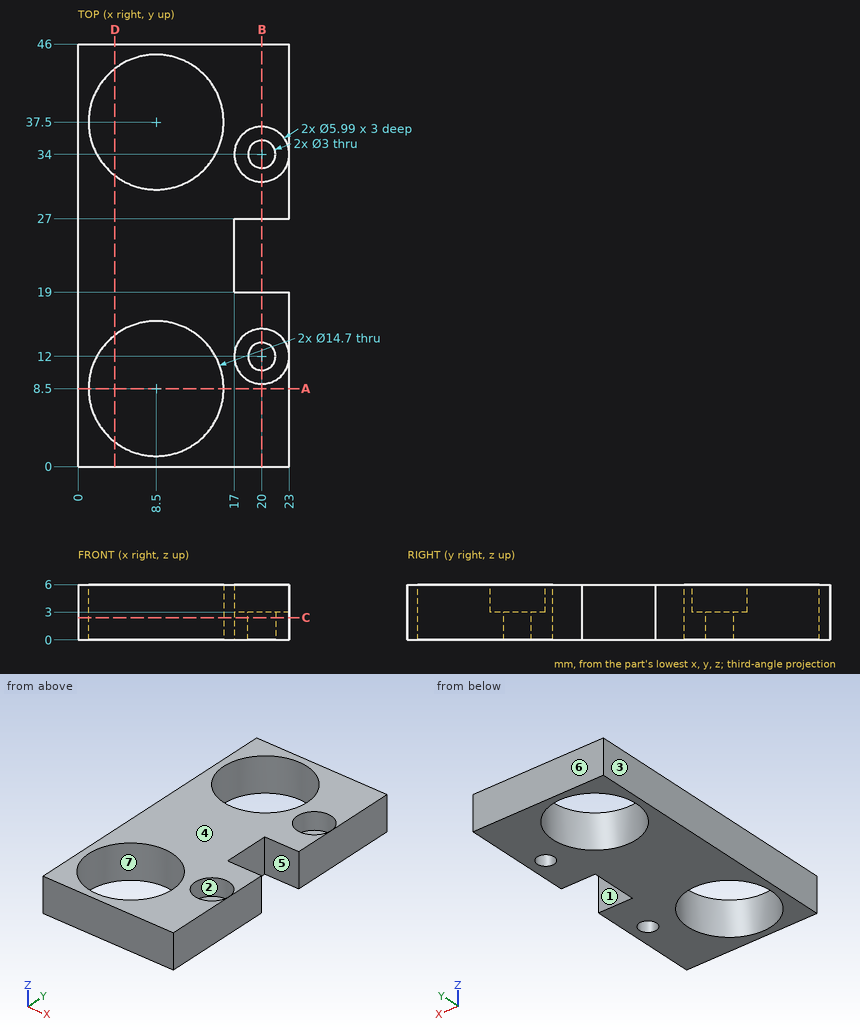
Here's the drawing with two shaded views (mm, measured from the low corner). I have some questions. A direction names the side the tool comes from. Coordinates: 2 decimals unless noted, no trailing zeros. Order: outer loops, then holes, each group sorted by start corner. A loop starts at its lowest first (then second) coordinate and runs counter-clockwise, first axis right, second up. Notation, with made-up numbers: (26.25, 41) - (45.25, 41) arc R30 ccw to (45.25, 76) - close; hole circle Ø10 at (5, 52). An arc over 180 degrees is marked (long way). Answer in a Markdown table with one row per item.
1. Suppose I cut it at C-C (z = 2.4). Please give me the cut outline in (x, y), and give its area (3 significant figures).
Reply:
| item | result |
|---|---|
| outline | (0, 0) - (23, 0) - (23, 19) - (17, 19) - (17, 27) - (23, 27) - (23, 46) - (0, 46) - close; hole circle Ø14.7 at (8.5, 8.5); hole circle Ø14.7 at (8.5, 37.5); hole circle Ø3 at (20, 12); hole circle Ø3 at (20, 34) |
| area | 656 mm^2 |
2. Suppose I cut it at B-B (x = 20). Please give me the cut outline in (y, z) (3 decimals).
Reply:
| item | result |
|---|---|
| outline | (0, 0) - (10.5, 0) - (10.5, 3) - (9.005, 3) - (9.005, 6) - (0, 6) - close; (13.5, 0) - (19, 0) - (19, 6) - (14.995, 6) - (14.995, 3) - (13.5, 3) - close; (27, 0) - (32.5, 0) - (32.5, 3) - (31.005, 3) - (31.005, 6) - (27, 6) - close; (35.5, 0) - (46, 0) - (46, 6) - (36.995, 6) - (36.995, 3) - (35.5, 3) - close |
3. Suppose I cut it at D-D (x = 4). Please give me the cut outline in (y, z).
Reply:
| item | result |
|---|---|
| outline | (0, 0) - (2.69, 0) - (2.69, 6) - (0, 6) - close; (14.31, 0) - (31.69, 0) - (31.69, 6) - (14.31, 6) - close; (43.31, 0) - (46, 0) - (46, 6) - (43.31, 6) - close |
4. If we mould it in two halves opening along Y, with no side actions, what happens to the marked faces 4, 5, 6 and 7? For each: pulls with the +Y half, pulls with the -Y half, needs draft (parallel to the pull), parting line crosses it, or undercut.
Reply:
| item | result |
|---|---|
| face 4 | needs draft |
| face 5 | undercut |
| face 6 | pulls with the +Y half |
| face 7 | undercut |
5. Suppose I cut it at A-A (y = 8.5). Please give me the cut outline in (x, z), and give its area (3 significant figures).
Reply:
| item | result |
|---|---|
| outline | (0, 0) - (1.15, 0) - (1.15, 6) - (0, 6) - close; (15.85, 0) - (23, 0) - (23, 6) - (15.85, 6) - close |
| area | 49.8 mm^2 |
6. For the marked faces 1, 2 and 3, which set-ups out of +Z, -Z, +X, -X, +Y, -Y let a thin tool reach every point of the face, with its end or its side?
Reply:
| item | result |
|---|---|
| face 1 | +Z, -Z, +X |
| face 2 | +Z |
| face 3 | +Z, -Z, -X, +Y, -Y |
7. If I drill on line 1 along Y through (x, z) = (20, 2); line 2 along Y through (x, z) = (4.5, 3.15); line 3 along Y through (x, z) = (8, 4), over which ranges is the centre line in solid material (lowest first)?
Reply:
| item | result |
|---|---|
| line 1 | y = 0 to 10.5, 13.5 to 19, 27 to 32.5, 35.5 to 46 |
| line 2 | y = 0 to 2.33, 14.67 to 31.33, 43.67 to 46 |
| line 3 | y = 0 to 1.17, 15.83 to 30.17, 44.83 to 46 |
